```python
from build123d import *

# Parameters (mm, degrees)
SKETCH_1_W          = 20
SKETCH_1_H          = 18
EXTRUDE_1_DEPTH     = 15
SKETCH_2_R          = 1.5
CUT_EXTRUDE_1_DEPTH = 31.805843601
SKETCH_3_W          = 10
SKETCH_3_H          = 10
CUT_EXTRUDE_2_DEPTH = 15
SKETCH_5_W          = 4
SKETCH_5_H          = 18
CUT_EXTRUDE_3_DEPTH = 31.805843601
SKETCH_6_R          = 1
CUT_EXTRUDE_4_DEPTH = 30.068883707
SKETCH_8_W          = 11.4
SKETCH_8_H          = 10
CUT_EXTRUDE_5_DEPTH = 10
SKETCH_9_W          = 11.4
SKETCH_9_H          = 10
EXTRUDE_2_DEPTH     = 7
SKETCH_10_R         = 1.075
CUT_EXTRUDE_6_DEPTH = 20
SKETCH_11_W         = 5
SKETCH_11_H         = 18
CUT_EXTRUDE_7_DEPTH = 20
SKETCH_12_W         = 9
SKETCH_12_H         = 10
CUT_EXTRUDE_8_DEPTH = 20
FILLET_1_R          = 2
FILLET_2_R          = 2
FILLET_3_R          = 2
FILLET_4_R          = 2
FILLET_5_R          = 2
FILLET_6_R          = 2


with BuildPart() as part:
    # 草图1 → 凸台-拉伸1 (new body)
    with BuildSketch(Plane.XY):
        with Locations((10, 9)):
            Rectangle(SKETCH_1_W, SKETCH_1_H)
    extrude(amount=EXTRUDE_1_DEPTH)

    # 草图2 → 切除-拉伸1 (cut, through all)
    with BuildSketch(Plane(origin=(20, 0, 0), x_dir=(0, 0, -1), z_dir=(1, 0, 0))):
        with Locations(Location((-7.5, 3, 0), (0, 0, 90))):
            Circle(SKETCH_2_R)
        with Locations((-7.5, 22)):
            Circle(SKETCH_2_R)
    extrude(amount=-CUT_EXTRUDE_1_DEPTH, mode=Mode.SUBTRACT)

    # 草图3 → 切除-拉伸2 (cut)
    with BuildSketch(Plane.XY.offset(15)):
        with Locations((10, 13)):
            Rectangle(SKETCH_3_W, SKETCH_3_H)
    extrude(amount=-CUT_EXTRUDE_2_DEPTH, mode=Mode.SUBTRACT)

    # 草图5 → 切除-拉伸3 (cut, through all)
    with BuildSketch(Plane(origin=(20, 0, 0), x_dir=(0, 0, -1), z_dir=(1, 0, 0))):
        with Locations((-13, 9)):
            Rectangle(SKETCH_5_W, SKETCH_5_H)
        with Locations((-2, 9)):
            Rectangle(SKETCH_5_W, SKETCH_5_H)
    extrude(amount=-CUT_EXTRUDE_3_DEPTH, mode=Mode.SUBTRACT)

    # 草图6 → 切除-拉伸4 (cut, through all)
    with BuildSketch(Plane(origin=(20, 0, 0), x_dir=(0, 0, -1), z_dir=(1, 0, 0))):
        with Locations(Location((-7.5, 15, 0), (0, 0, 90))):
            Circle(SKETCH_6_R)
    extrude(amount=-CUT_EXTRUDE_4_DEPTH, mode=Mode.SUBTRACT)

    # 草图8 → 切除-拉伸5 (cut)
    with BuildSketch(Plane.XY.offset(11)):
        with Locations((10, 13)):
            Rectangle(SKETCH_8_W, SKETCH_8_H)
    extrude(amount=-CUT_EXTRUDE_5_DEPTH, mode=Mode.SUBTRACT)

    # 草图9 → 凸台-拉伸2 (add)
    with BuildSketch(Plane.XY.offset(11)):
        with Locations((10, 13)):
            Rectangle(SKETCH_9_W, SKETCH_9_H)
    extrude(amount=-EXTRUDE_2_DEPTH)

    # 草图10 → 切除-拉伸6 (cut)
    with BuildSketch(Plane(origin=(20, 0, 0), x_dir=(0, 0, -1), z_dir=(1, 0, 0))):
        with Locations(Location((-7.5, 15, 0), (0, 0, 90))):
            Circle(SKETCH_10_R)
    extrude(amount=-CUT_EXTRUDE_6_DEPTH, mode=Mode.SUBTRACT)

    # 草图11 → 切除-拉伸7 (cut)
    with BuildSketch(Plane.XY.offset(11)):
        with Locations((17.5, 9)):
            Rectangle(SKETCH_11_W, SKETCH_11_H)
    extrude(amount=-CUT_EXTRUDE_7_DEPTH, mode=Mode.SUBTRACT)

    # 草图12 → 切除-拉伸8 (cut)
    with BuildSketch(Plane.XY.offset(11)):
        with Locations((7.5, 13)):
            Rectangle(SKETCH_12_W, SKETCH_12_H)
    extrude(amount=-CUT_EXTRUDE_8_DEPTH, mode=Mode.SUBTRACT)

    # 圆角1
    fillet_1_edges = [part.edges().sort_by_distance(p)[0] for p in [
        (7.5, 0, 11),
    ]]
    fillet(fillet_1_edges, radius=FILLET_1_R)

    # 圆角2
    fillet_2_edges = [part.edges().sort_by_distance(p)[0] for p in [
        (7.5, 0, 4),
    ]]
    fillet(fillet_2_edges, radius=FILLET_2_R)

    # 圆角3
    fillet_3_edges = [part.edges().sort_by_distance(p)[0] for p in [
        (1.5, 18, 11),
    ]]
    fillet(fillet_3_edges, radius=FILLET_3_R)

    # 圆角4
    fillet_4_edges = [part.edges().sort_by_distance(p)[0] for p in [
        (13.5, 18, 11),
    ]]
    fillet(fillet_4_edges, radius=FILLET_4_R)

    # 圆角5
    fillet_5_edges = [part.edges().sort_by_distance(p)[0] for p in [
        (13.5, 18, 4),
    ]]
    fillet(fillet_5_edges, radius=FILLET_5_R)

    # 圆角6
    fillet_6_edges = [part.edges().sort_by_distance(p)[0] for p in [
        (1.5, 18, 4),
    ]]
    fillet(fillet_6_edges, radius=FILLET_6_R)


solid = part.part
```
Read the model definition and answer for the solid it produces. Units are mm, in the model's axes. A direction names the side the tool comes from. Give positions to 0.01 mm unless a question says otherwise; leave off trailing zeros. Order: outer loops, then holes, each group sorted by start corner. A loop starts at its lowest first (then second) coordinate and runs counter-clockwise, first axis right, second up. Notation, with made-up numbers: (48, 63.25) -> (72, 63.25) arc R38 cw to (72, 101.25) -> close; hole circle Ø7 at (-25.5, 14). An arc over 180 degrees is marked (long way). Write item = value, one per line.
1. A cutting plane is placed at B-B, the plane y = 15. Write down the section's boundary in (x, z) (3 decimals), and give its area (3 significant figures).
Numbers:
outline = (0, 4) -> (3, 4) -> (3, 6.425) -> (0, 6.425) -> close; (0, 8.575) -> (3, 8.575) -> (3, 11) -> (0, 11) -> close; (12, 4) -> (15, 4) -> (15, 6.425) -> (12, 6.425) -> close; (12, 8.575) -> (15, 8.575) -> (15, 11) -> (12, 11) -> close
area = 29.1 mm²
2. Given pin 1 (2 mm diameter, centred on x = 10, z = 8.5, fed in from +Y); pin 2 (3 mm diameter, centred on y = 6, z = 6, fed in from -X); pin 3 (1.8 mm diameter, centred on y = 3, z = 7.5, fed in from +X), each flat-ended and moving along its own axis, determine where each tip first touches the part or whether it passes through.
Numbers:
pin_1 = 8
pin_2 = 0
pin_3 = through
3. The mould has two halves that part along Y. Classify faces 1 (the face through (0, 9, 7)), 2 (the face through (13.52, 17.43, 4.6)), 3 (the face through (1.52, 15.5, 6.55)): +Y half, -Y half, draft (parallel to the pull), parting line (faces both ways), or undercut.
Numbers:
face_1 = draft
face_2 = +Y half
face_3 = undercut
4. A cutting plane is placed at C-C, the plane x = 10.5. Write down the section's boundary in (y, z), and give its area (3 significant figures).
Numbers:
outline = (0, 6) arc R2 ccw to (2, 4) -> (8, 4) -> (8, 11) -> (2, 11) arc R2 ccw to (0, 9) -> close; hole circle Ø3 at (3, 7.5)
area = 47.2 mm²
5. Straight lines are drawn through the part: line 1 along Z through (x, y) = (1.7, 15) (3 decimals); line 2 along X through (y, z) = (16, 9); line 3 along Z through (x, y) = (5.75, 3). For each, find the intervals that lie inside material, in ascending order.
Numbers:
line_1 = 4 to 6.425, 8.575 to 11
line_2 = 0 to 3, 12 to 15
line_3 = 4 to 6, 9 to 11
6. A cutting plane is placed at A-A, the plane y = 3. Write down the section's boundary in (x, z), and give its area (3 significant figures).
Numbers:
outline = (0, 4) -> (15, 4) -> (15, 6) -> (0, 6) -> close; (0, 9) -> (15, 9) -> (15, 11) -> (0, 11) -> close
area = 60.0 mm²
7. For faces 4 (the face through (7.4, 0.57, 10.4)), 5 (the face through (12, 13, 8)), determine the directions among +Z, -Z, +X, -X, +Y, -Y from which every point of the face is accessible in a straight line to the end or side of a thin tool.
Numbers:
face_4 = +Z, +X, -X, -Y
face_5 = +Z, -Z, +Y
8. A cutting plane is placed at D-D, the plane z = 7.5. Write down the section's boundary in (x, y) (3 decimals), and give its area (3 significant figures).
Numbers:
outline = (0, 0) -> (15, 0) -> (15, 1.5) -> (0, 1.5) -> close; (0, 4.5) -> (15, 4.5) -> (15, 13.925) -> (12, 13.925) -> (12, 8) -> (3, 8) -> (3, 13.925) -> (0, 13.925) -> close; (0, 16.075) -> (3, 16.075) -> (3, 18) -> (0, 18) -> close; (12, 16.075) -> (15, 16.075) -> (15, 18) -> (12, 18) -> close
area = 122 mm²
